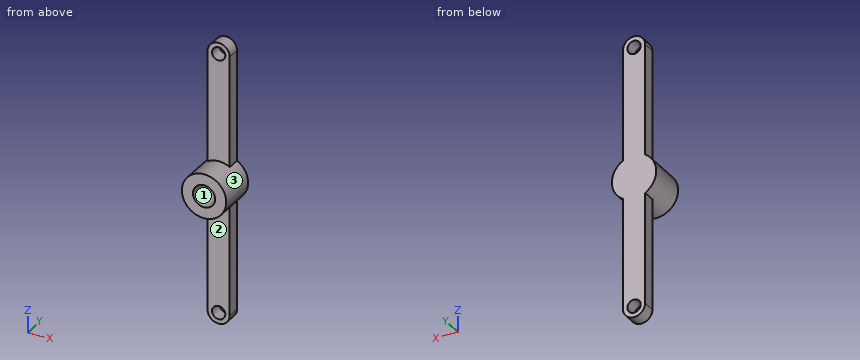
Autodesk Inventor part; units mm, degrees
ref_plane "YZ Plane" through (0, 0, 0) normal (1, 0, 0) x (0, 1, 0)
ref_plane "XZ Plane" through (0, 0, 0) normal (0, 1, 0) x (-1, 0, 0)
ref_plane "XY Plane" through (0, 0, 0) normal (0, 0, 1) x (1, 0, 0)
sketch "Sketch1" plane through (0, 0, 0) normal (0, 1, 0) x (-1, 0, 0)
  circle A0 centre (0, 0) radius 5
  line L0 (2.5, 4.3301) -> (2.5, -4.3301)
  line L1 (-2.5, 4.3301) -> (-2.5, -4.3301)
  line L2 (-2.5, 4.3301) -> (-2.5, -4.3301)
  line L3 (-2.5, 4.3301) -> (-2.5, 29.3301)
  line L4 (-2.5, -4.3301) -> (-2.5, -29.3301)
  line L5 (2.5, -4.3301) -> (2.5, -29.3301)
  arc A1 (-2.5, -29.3301) -> (2.5, -29.3301) centre (0, -29.3301) ccw
  line L6 (2.5, 4.3301) -> (2.5, 29.3301)
  arc A2 (2.5, 29.3301) -> (-2.5, 29.3301) centre (0, 29.3301) ccw
  circle A3 centre (0, 29.3301) radius 1.5
  circle A4 centre (0, -29.3301) radius 1.5
  dimension "d0" = 10
  dimension "d1" = 5
  dimension "d2" = 2.5
  dimension "d18" = 25
  dimension "d19" = 25
  dimension "d20" = 25
  dimension "d21" = 3
  dimension "d22" = 3
  dimension "d23" = 25
  dimension "d24" = 2.5
extrude "Extrusion1" add sketch "Sketch1" along normal blind 3
sketch "Sketch2" plane through (0, 0, 0) normal (0, -1, 0) x (1, 0, 0)
  circle A0 centre (0, 0) radius 5
  circle A1 centre (0, 0) radius 2.5
  dimension "d14" = 5
  dimension "d15" = 10
extrude "Extrusion2" add sketch "Sketch2" along normal blind 6
properties part number "gripper_mechanism"
The listing builds one solid part. Answer for the finished solid, in the listing's coordinates (mm). Face numbers are marked on the shaded views. Round coordinates to 2 decimals unless told otherwise and drop trailing zeros. Write each loop counter-clockwise with the first axis right and the second up, starting at its lowest first coordinate (ties: lowest second). Pieces come first, ordered by that corner, then holes. Notation, with made-up numbers: (18, -25) -> (51, -25) arc R15 cw to (51, -15) -> close; hole circle Ø10 at (-32.5, 0.25). An arc over 180 degrees is marked (long way). Use CSV: the item, a comma, the result in double quotes. Start each with the question number.
(1) Each of these flat-tipped pins is pushed along its axis until it touches: pin 1 (3 mm diameter, centred on y = 0, z = 3.5, fed in from +X); pin 2 (2.5 mm diameter, centred on y = 1, z = -15.5, fed in from +X); pin 3 (1.5 mm diameter, centred on x = -2, y = 2, fed in from +Z); pin 4 (2.5 mm diameter, centred on x = 0, z = -29.33, fed in from -Y). Where does it stop, or does it pass through?
(2) Consider L1, parallel to Z at x = 0, y = 2.1; L2, parallel to Z at x = 0, y = -3.5; L3, parallel to Z at x = -1.25, y = 2. Determine where each line is inside the solid, lowest interval first. Write a range as from..to.
(3) Section D-D on z = 12.5 is taken. Give the vertices of the cut face in (x, y), then the cut area to 3 significant figures.
(4) Section B-B on y = 1.75 is taken. Give the vertices of the cut face in (x, z).
(5) The mould has two halves that part along X. Classify the marked faces 1, 2 and 3: released by +X, released by -X, zero draft, split by the parting line, or undercut.
(6) Section C-C on y = -2 is taken. Give the vertices of the cut face in (x, z).
(7) Section A-A on x = 0 is taken. Give the vertices of the cut face in (y, z), then the cut area to 3 significant figures.
A:
1,pin 1,"stops at x = 4.58"
1,pin 2,"stops at x = 2.5"
1,pin 3,"stops at z = 31.5"
1,pin 4,"passes through"
2,L1,"z = -31.83..-30.83, -27.83..27.83, 30.83..31.83"
2,L2,"z = -5..-2.5, 2.5..5"
2,L3,"z = -31.5..-30.16, -28.5..28.5, 30.16..31.5"
3,outline,"(-2.5, 0) -> (2.5, 0) -> (2.5, 3) -> (-2.5, 3) -> close"
3,area,"15.0 mm²"
4,outline,"(-2.5, -29.33) arc R2.5 ccw to (2.5, -29.33) -> (2.5, -4.33) arc R5 ccw to (2.5, 4.33) -> (2.5, 29.33) arc R2.5 ccw to (-2.5, 29.33) -> (-2.5, 4.33) arc R5 ccw to (-2.5, -4.33) -> close; hole circle Ø3 at (0, -29.33); hole circle Ø3 at (0, 29.33)"
5,face 1,"undercut"
5,face 2,"zero draft"
5,face 3,"split by the parting line"
6,outline,"circle Ø10 at (0, 0); hole circle Ø5 at (0, 0)"
7,outline,"(-6, -5) -> (0, -5) -> (0, -27.83) -> (3, -27.83) -> (3, 27.83) -> (0, 27.83) -> (0, 5) -> (-6, 5) -> (-6, 2.5) -> (0, 2.5) -> (0, -2.5) -> (-6, -2.5) -> close; (0, -31.83) -> (3, -31.83) -> (3, -30.83) -> (0, -30.83) -> close; (0, 30.83) -> (3, 30.83) -> (3, 31.83) -> (0, 31.83) -> close"
7,area,"203 mm²"
